Source: three-view drawing plus pictorial views. Frame: mm from the lowest corner of the part. A direction names the side the tool comes from. Round coordinates to 2 decimals unless told otherwise and drop trailing zeros. Loops run counter-clockwise (first coordinate to the right, second up) from the corner with the lowest first, then second, coordinate; pieces in that order, holes last. Notation, with made-up numbers: M 32,-29 L 71,-29 A28 cw 71,2 Z; hole C 76,16.25 d1. An arc over 180 degrees is marked long. Answer as a JSON object with one key per item and string values.
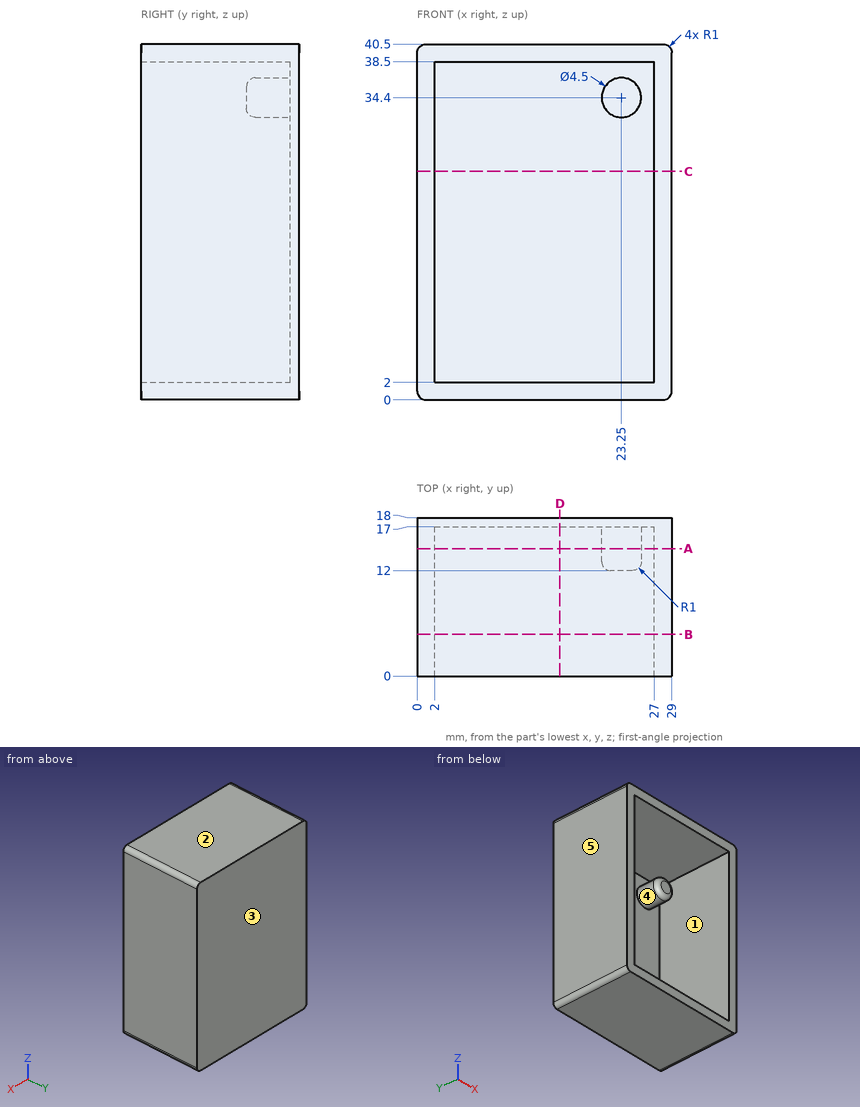
1) Pull-direction query (Z, two-part tool) for the marked faces 1, 2 and 3; classes: +Z half, -Z half, draft (parallel to the pull), parting line (faces both ways), or undercut.
Geometry results:
{"face 1": "undercut", "face 2": "+Z half", "face 3": "draft"}
2) First-contact query: pin 1 (1.2 mm diameter, centred on x = 23.5, z = 35, fed in from -Y). Flat tip, straight axial feed; report the tip coordinate or a pass-through.
Geometry results:
{"pin 1": "y = 12"}
3) Cut plane B-B on y = 4.75. Return the cut outline in (x, z), and give its area (3 significant figures).
Geometry results:
{"outline": "M 0,1 A1 ccw 1,0 L 28,0 A1 ccw 29,1 L 29,39.5 A1 ccw 28,40.5 L 1,40.5 A1 ccw 0,39.5 Z; hole M 2,2 L 27,2 L 27,38.5 L 2,38.5 Z", "area": "261 mm2"}
4) Cut plane A-A on y = 14.5. Return the cut outline in (x, z), and give its area (3 significant figures).
Geometry results:
{"outline": "M 0,1 A1 ccw 1,0 L 28,0 A1 ccw 29,1 L 29,39.5 A1 ccw 28,40.5 L 1,40.5 A1 ccw 0,39.5 Z; C 23.25,34.4 d4.5; hole M 2,2 L 27,2 L 27,38.5 L 2,38.5 Z", "area": "277 mm2"}
5) Set-up query: the marked faces 4 and 5. Return all of +Z, -Z, +X, -X, +Y, -Y with unobstructed straight access to the full face (end or side cutting, diameter ignored); none if empty.
Geometry results:
{"face 4": "-Y", "face 5": "+Z, -Z, -X, +Y, -Y"}
6) Line query: probe 1 along Z at (x, y) = (15.25, 8.5); probe 2 along X at (y, z) = (15.75, 12); probe 3 along Y at (x, z) = (15.5, 26). Output: solid intervals per line, ascending.
Geometry results:
{"probe 1": "0 to 2, 38.5 to 40.5", "probe 2": "0 to 2, 27 to 29", "probe 3": "17 to 18"}
7) Cut plane C-C on z = 26. Return the cut outline in (x, y), and give its area (3 significant figures).
Geometry results:
{"outline": "M 0,0 L 2,0 L 2,17 L 27,17 L 27,0 L 29,0 L 29,18 L 0,18 Z", "area": "97.0 mm2"}
8) Cut plane D-D on x = 16.25. Return the cut outline in (y, z).
Geometry results:
{"outline": "M 0,0 L 18,0 L 18,40.5 L 0,40.5 L 0,38.5 L 17,38.5 L 17,2 L 0,2 Z"}
